For this review, take the finished solid that the model builds, in its own axes (mm). Face numbers are marked on the shaded views. A direction names the side the tool comes from. Give positions to 0.01 mm unless a question says otherwise; leave off trailing zeros. Order: outer loops, then holes, each group sorted by start corner. A loop starts at its lowest first (then second) coordinate and runs counter-clockwise, first axis right, second up. Notation, with made-up numbers: (20, 79.5) - (70, 79.5) arc R21 cw to (70, 94.5) - close; hole circle Ø5 at (70, 39.25). An arc over 180 degrees is marked (long way). One line per item, written item: value.
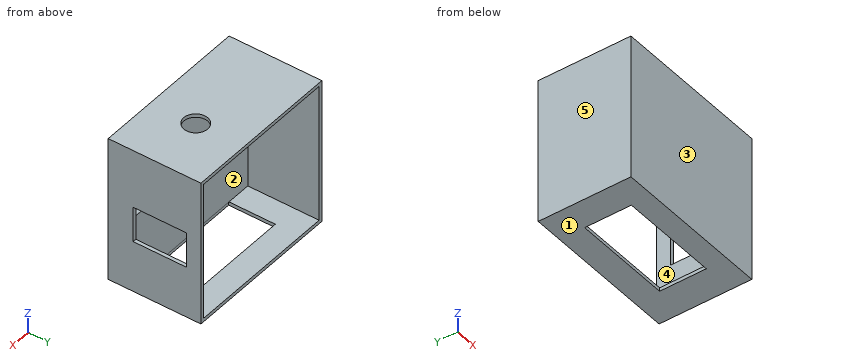
Autodesk Inventor part; units mm, degrees
ref_plane "YZ Plane" through (0, 0, 0) normal (1, 0, 0) x (0, 1, 0)
ref_plane "XZ Plane" through (0, 0, 0) normal (0, 1, 0) x (-1, 0, 0)
ref_plane "XY Plane" through (0, 0, 0) normal (0, 0, 1) x (1, 0, 0)
sketch "Szkic1" plane through (0, 0, 0) normal (0, 1, 0) x (-1, 0, 0)
  line L0 (0, 0) -> (45, 0)
  line L1 (45, 0) -> (45, -41)
  line L2 (45, -41) -> (0, -41)
  line L3 (0, -41) -> (0, 0)
  line L4 (45, 0) -> (44, 0)
  line L5 (44, 0) -> (44, -1)
  line L6 (0, -41) -> (0, -40)
  line L7 (0, -40) -> (1, -40)
  line L8 (1, -40) -> (44, -40)
  line L9 (44, -40) -> (44, -1)
  line L10 (44, -1) -> (1, -1)
  line L11 (1, -1) -> (1, -40)
  dimension "d0" = 45
  dimension "d1" = 41
  dimension "d2" = 1
  dimension "d3" = 1
  dimension "d4" = 1
  dimension "d5" = 1
extrude "Wyciągnięcie proste1" add sketch "Szkic1" along normal blind 18 contours L0 L5 L10 L11 L7 L3 | L0 L1 L2 L3 L7 L8 L9 L5
sketch "Szkic2" plane through (0, 0, -41) normal (0, 0, -1) x (-1, 0, 0)
  line L0 (40, 15) -> (12.1, 15)
  line L1 (12.1, 15) -> (12.1, 1.9)
  line L2 (12.1, 1.9) -> (40, 1.9)
  line L3 (40, 1.9) -> (40, 15)
  line L4 (40, 8.45) -> (38, 8.45)
  line L5 (12.1, 8.45) -> (10.1, 8.45)
  line L6 (10.1, 8.45) -> (38, 8.45)
  line L7 (38, 8.45) -> (38, 15)
  line L8 (38, 15) -> (10.1, 15)
  line L9 (10.1, 15) -> (10.1, 8.45)
  line L10 (38, 8.45) -> (10.1, 8.45)
  line L11 (10.1, 8.45) -> (10.1, 1.9)
  line L12 (10.1, 1.9) -> (38, 1.9)
  line L13 (38, 1.9) -> (38, 8.45)
  line L14 (10.1, 1.9) -> (9.1, 1.9)
  line L15 (9.1, 1.9) -> (9.1, 15)
  line L16 (9.1, 15) -> (10.1, 15)
  line L17 (10.1, 15) -> (10.1, 1.9)
  line L18 (38, 1.9) -> (37, 1.9)
  line L19 (37, 1.9) -> (37, 15)
  line L20 (37, 15) -> (38, 15)
  line L21 (38, 15) -> (38, 1.9)
  point P0 (0, 0)
  point P1 (10.1, 15)
  dimension "d8" = 27.9
  dimension "d9" = 13.1
  dimension "d33" = 2
  dimension "d34" = 2
  dimension "d35" = 1
  dimension "d36" = 1
extrude "Wyciągnięcie proste2" cut sketch "Szkic2" against normal blind 5.25 contours L19 L6 L1 L0 | L1 L5 L9 L8 | L19 L2 L1 L6 | L1 L12 L11 L5 | L9 L11 L14 L15 L16
sketch "Szkic3" plane through (0, 0, -41) normal (0, 0, -1) x (-1, 0, 0)
  line L0 (12.1, 1.9) -> (12.1, 15)
  line L1 (12.1, 8.45) -> (21.9, 8.45)
  line L2 (21.9, 8.45) -> (19.05, 8.45)
  circle A0 centre (19.05, 8.45) radius 3.35
  line L3 (19.05, 8.45) -> (16.05, 8.45)
  circle A1 centre (16.05, 8.45) radius 3.35
  point P0 (0, 0)
  dimension "d12" = 9.8
  dimension "d13" = 2.85
  dimension "d14" = 6.7
  dimension "d37" = 3
  dimension "d38" = 6.7
extrude "Wyciągnięcie proste3" cut sketch "Szkic3" against normal blind 48.25 contours L1 A0 A1 | L1 A1 A0 | A0 A1 L1 | L1 A1 A0
sketch "Szkic4" plane through (0, 0, 0) normal (1, 0, 0) x (0, 0, -1)
  line L0 (1, 18) -> (40, 18)
  line L1 (20.5, 18) -> (26.5, 18)
  line L2 (26.5, 18) -> (26.5, 3)
  line L3 (26.5, 3) -> (20.5, 3)
  line L4 (20.5, 3) -> (20.5, 18)
  line L5 (20.5, 18) -> (16.5, 18)
  line L6 (16.5, 18) -> (16.5, 3)
  line L7 (16.5, 3) -> (20.5, 3)
  line L8 (20.5, 3) -> (20.5, 18)
  point P0 (0, 0)
  dimension "d17" = 6
  dimension "d18" = 15
  dimension "d19" = 4
extrude "Wyciągnięcie proste4" cut sketch "Szkic4" against normal blind 24.25
sketch "Szkic5" plane through (0, 0, 0) normal (0, -1, 0) x (1, 0, 0)
  line L0 (-1, -40) -> (-1, -26.5)
  line L1 (-44, -1) -> (-44, -40)
  line L2 (-1, -40) -> (-44, -40)
  line L3 (-44, -40) -> (-44, -21)
  line L4 (-44, -21) -> (-1, -21)
  line L5 (-1, -21) -> (-1, -40)
  line L6 (0, 0) -> (0, -41)
  line L7 (0, -41) -> (-45, -41)
  line L8 (0, -21) -> (-45, -21)
  line L9 (-45, -21) -> (-45, -41)
  line L10 (-45, -41) -> (0, -41)
  line L11 (0, -41) -> (0, -21)
  dimension "d22" = 19
extrude "Wyciągnięcie proste5" add sketch "Szkic5" against normal blind 2 contours L2 L1 L4 L5 L0
sketch "Szkic6" plane through (0, 0, 0) normal (0, -1, 0) x (1, 0, 0)
  line L0 (0, 0) -> (-45, 0)
  line L1 (-45, 0) -> (-45, -40.9786)
  line L2 (-45, -40.9786) -> (0, -40.9786)
  line L3 (0, -40.9786) -> (0, 0)
extrude "Wyciągnięcie proste6" add sketch "Szkic6" along normal blind 4
sketch "Szkic7" plane through (0, 0, 0) normal (0, 1, 0) x (1, 0, 0)
  line L0 (-1, 1) -> (-44, 1)
  line L1 (-44, 21) -> (-1, 21)
  line L2 (-44, 1) -> (-1, 1)
  line L3 (-1, 1) -> (-1, 21)
  line L4 (-1, 21) -> (-44, 21)
  line L5 (-44, 21) -> (-44, 1)
  point P0 (0, 0)
extrude "Wyciągnięcie proste7" cut sketch "Szkic7" against normal blind 2
sketch "Szkic8" plane through (0, 0, -40.9786) normal (0, 0, -1) x (-1, 0, 0)
  line L0 (45, -4) -> (0, -4)
  line L1 (0, 0) -> (45, 0)
  line L2 (45, -4) -> (0, -4)
  line L3 (0, -4) -> (0, 0)
  line L4 (0, 0) -> (45, 0)
  line L5 (45, 0) -> (45, -4)
extrude "Wyciągnięcie proste8" add sketch "Szkic8" along normal blind 0.0214
sketch "Szkic9" plane through (0, 18, 0) normal (0, 1, 0) x (1, 0, 0)
  line L0 (0, 26.5) -> (0, 41)
  line L1 (0, 0) -> (-45, 0)
  line L2 (0, 41) -> (-45, 41)
  line L3 (-45, 41) -> (-45, 0)
  line L4 (-45, 0) -> (0, 0)
  line L5 (0, 0) -> (0, 41)
  line L6 (-1, 40) -> (-1, 26.5)
  line L7 (-44, 1) -> (-44, 40)
  line L8 (-1, 40) -> (-44, 40)
  line L9 (-44, 40) -> (-44, 1)
  line L10 (-44, 1) -> (-1, 1)
  line L11 (-1, 1) -> (-1, 40)
extrude "Wyciągnięcie proste9" add sketch "Szkic9" along normal blind 4
sketch "Szkic10" plane through (0, -4, -41) normal (0, 0, -1) x (-1, 0, 0)
  circle A0 centre (16.05, 12.45) radius 3.35
  circle A1 centre (16.05, 12.45) radius 3.35
  point P0 (0, 4)
(1) Take a section at A-A (x = -30). Write out the cut boundary in (y, z).
Answers below:
outline: (-4, -41) - (1.9, -41) - (1.9, -40) - (2, -40) - (2, -21) - (-2, -21) - (-2, -1) - (22, -1) - (22, 0) - (-4, 0) - close; (15, -41) - (22, -41) - (22, -40) - (15, -40) - close
(2) For P1, Ø4, axis at x = -26.5, z = -24, coming from the +Y side; P2, Ø6, axis at x = -16.05, y = 8.45, coming from the -Z side, all flat-tipped, find the tip position at first contact; note any pin that passes through.
Answers below:
P1: stops at y = 2
P2: passes through
(3) Draft analysis for pull direction X (two halves, no side actions). For the marked faces 3, 4 and 5, state which applies: pulls with the +X half, pulls with the -X half, needs draft (parallel to the pull), parting line crosses it, or undercut.
Answers below:
face 3: needs draft
face 4: undercut
face 5: pulls with the -X half
(4) Machinability: for the marked faces 1 and 2, which of the approach directions +Z, -Z, +X, -X, +Y, -Y give a long, thin tool a straight path to every point of the face, cutting with its end or side? Answer none if there is none.
Answers below:
face 1: -Z, +X, -X, +Y, -Y
face 2: +Y
(5) Wall thickness on line 1 (Y direction, x = -16.05, z = -0.6); line 2 (X direction, y = 20.25, z = -19.5); line 3 (Z direction, x = -4.5, y = 21.25): over which ranges is each line inside the solid? List them lowest first. Write a range as from..to.
Answers below:
line 1: y = -4..5.1, 11.8..22
line 2: x = -45..-44, -1..0
line 3: z = -41..-40, -1..0
(6) Take a section at D-D (x = -16.05). Write out the cut boundary in (y, z), then the cut area to 3 significant figures.
Answers below:
outline: (-4, -41) - (1.9, -41) - (1.9, -40) - (2, -40) - (2, -21) - (-2, -21) - (-2, -1) - (5.1, -1) - (5.1, 0) - (-4, 0) - close; (11.8, -1) - (22, -1) - (22, 0) - (11.8, 0) - close; (15, -41) - (22, -41) - (22, -40) - (15, -40) - close
area: 186 mm^2
(7) Take a section at C-C (z = -18.5). Write out the cut boundary in (x, y), then the cut area to 3 significant figures.
Answers below:
outline: (-45, -4) - (0, -4) - (0, 3) - (-1, 3) - (-1, -2) - (-44, -2) - (-44, 22) - (-45, 22) - close; (-1, 18) - (0, 18) - (0, 22) - (-1, 22) - close
area: 123 mm^2
(8) Take a section at B-B (y = 8.45). Write out the cut boundary in (x, z), then the cut area to 3 significant figures.
Answers below:
outline: (-45, -41) - (-37, -41) - (-37, -40) - (-44, -40) - (-44, -1) - (-19.4, -1) - (-19.4, 0) - (-45, 0) - close; (-12.7, -1) - (-1, -1) - (-1, -16.5) - (0, -16.5) - (0, 0) - (-12.7, 0) - close; (-9.1, -41) - (0, -41) - (0, -26.5) - (-1, -26.5) - (-1, -40) - (-9.1, -40) - close
area: 123 mm^2
